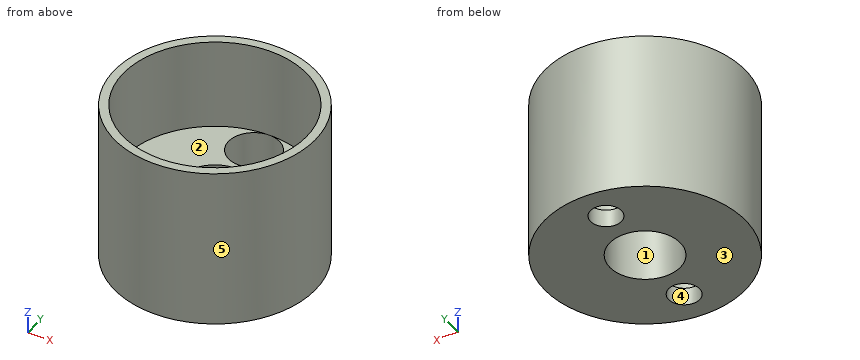
Autodesk Inventor part; units mm, degrees
ref_plane "Work Plane1" through (-9.0805, -9.0805, 27.1559) normal (0, 0, -1) x (0.0062, 1, 0)
ref_plane "YZ Plane" through (0, 0, 0) normal (1, 0, 0) x (0, 1, 0)
ref_plane "XZ Plane" through (0, 0, 0) normal (0, 1, 0) x (-1, 0, 0)
sketch "Sketch1" plane through (0, 0, 0) normal (0, 0, 1) x (1, 0, 0)
  circle A0 centre (0, 0) radius 9.025
  dimension "d0" = 18.05
extrude "Extrusion1" add sketch "Sketch1" along normal blind 6.35
sketch "Sketch4" plane through (0, 0, 6.35) normal (0, 0, 1) x (1, 0, 0)
  circle A0 centre (0, 0) radius 3.175
  dimension "d6" = 6.35
sketch "Sketch6" plane through (0, 0, 6.35) normal (0, 0, 1) x (1, 0, 0)
  circle A0 centre (0, 0) radius 9.025
  circle A1 centre (0, 0) radius 8.2312
  circle A2 centre (0, 0) radius 9.025
  dimension "d11" = 0.7937
ref_plane "Work Plane1" through (-9.0805, -9.0805, 27.1559) normal (0, 0, -1) x (0.0062, 1, 0)
extrude "Extrusion3" add sketch "Sketch6" along normal up to surface (20.8059 mm away)
sketch "Sketch7" plane through (0, 0, 6.35) normal (0, 0, 1) x (1, 0, 0)
  circle A0 centre (0, 5.9436) radius 1.397
  circle A1 centre (0, -5.9436) radius 1.397
  circle A2 centre (0, 0) radius 8.2312
  dimension "d20" = 2.794
  dimension "d21" = 2.794
  dimension "d22" = 5.9436
  dimension "d23" = 5.9436
extrude "Extrusion4" cut sketch "Sketch7" against normal blind 25.4 contours A0 | A1
sketch "Sketch8" plane through (0, 0, 6.35) normal (0, 0, 1) x (1, 0, 0)
  circle A0 centre (0, 5.9436) radius 2.286
  circle A1 centre (0, -5.9436) radius 2.286
  circle A2 centre (0, 5.9436) radius 1.397
  circle A3 centre (0, -5.9436) radius 1.397
  point P0 (0, 0)
  dimension "d16" = 4.572
  dimension "d17" = 4.572
extrude "Extrusion5" cut sketch "Sketch8" against normal blind 4.7625 contours A0 | A1 | A2 | A3
extrude "Extrusion6" cut sketch "Sketch4" against normal blind 25.4
sketch "Sketch9" plane through (0, 0, 27.1559) normal (0, 0, 1) x (1, 0, 0)
  circle A0 centre (27.8867, -20.1987) radius 65.8542
  point P0 (0, 0)
extrude "Extrusion7" cut sketch "Sketch9" against normal blind 12.7
properties part number "Cap Cap no LED"
Could you check a few things on this model? Use its own coordinates, in mm. Face numbers are marked on the shaded views. A direction names the side the tool comes from. Coordinates: 2 decimals unless noted, no trailing zeros. Write each loop counter-clockwise with the first axis right and the second up, starting at its lowest first coordinate (ties: lowest second). Pieces come first, ordered by that corner, then holes. Notation, with made-up numbers: (76.25, 77.5) -> (128.25, 77.5) arc R33 cw to (128.25, 105.5) -> close; hole circle Ø1 at (14, 42.25). An arc over 180 degrees is marked (long way). Write item = value, one per line. Start each with the question number.
(1) Will these pins go through, and if not, where does the flat tip stop? pin 1 (3 mm diameter, centred on y = 3, z = 5, fed in from +X); pin 2 (2.5 mm diameter, centred on x = 0, y = -5.94, fed in from +Z); pin 3 (3.5 mm diameter, centred on x = -0.5, y = -6.5, fed in from +Z); pin 4 (1.5 mm diameter, centred on x = 7, z = 5, fed in from -Y).
(2) We'd pull the mould along X, two halves only. Please class the marked faces 3, 4 and 5: released by +X, released by -X, zero draft, split by the parting line, or undercut.
(3) I want a section at A-A (y = 0). Please give me the cut outline in (x, z) (3 decimals).
(4) I want a section at B-B (x = 0). Give the number of separate pieces and of enclosed holes in the cut face, plus the area to 3 significant figures.
(5) I want a section at D-D (y = -5). Please give me the cut outline in (x, z), plus the area to 3 significant figures.
(6) Which directions (+Z, -Z, +X, -X, +Y, -Y) give clear straight access to the entire face, cutting with the end or side of a thin tool? Please do the marked faces 1 and 2.
(7) I want a section at C-C (z = 7). Please give me the cut outline in (x, y) (3 decimals), plus the area to 3 significant figures.
(8) I need wall thicknesses on line 1 (Y direction, x = 0, z = 5) (3 decimals); line 2 (Y direction, x = 0, z = 9) (3 decimals); line 3 (X direction, y = -0.25, z = 10.5). Which ranges of each line are inside material? Lowest first, please. Write a range as [from, to].
Result set:
q1.pin_1 = 8.9
q1.pin_2 = through
q1.pin_3 = 14.46
q1.pin_4 = -6.51
q2.face_3 = zero draft
q2.face_4 = undercut
q2.face_5 = split by the parting line
q3.outline = (-9.025, 0) -> (-3.175, 0) -> (-3.175, 6.35) -> (-8.231, 6.35) -> (-8.231, 14.456) -> (-9.025, 14.456) -> close; (3.175, 0) -> (9.025, 0) -> (9.025, 14.456) -> (8.231, 14.456) -> (8.231, 6.35) -> (3.175, 6.35) -> close
q4.separate_pieces = 4
q4.enclosed_holes = 0
q4.area = 34.7 mm2
q5.outline = (-7.51, 0) -> (-1.03, 0) -> (-1.03, 1.59) -> (-2.08, 1.59) -> (-2.08, 6.35) -> (-6.54, 6.35) -> (-6.54, 14.46) -> (-7.51, 14.46) -> close; (1.03, 0) -> (7.51, 0) -> (7.51, 14.46) -> (6.54, 14.46) -> (6.54, 6.35) -> (2.08, 6.35) -> (2.08, 1.59) -> (1.03, 1.59) -> close
q5.area = 88.1 mm2
q6.face_1 = +Z, -Z
q6.face_2 = +Z
q7.outline = circle Ø18.05 at (0, 0); hole circle Ø16.462 at (0, 0)
q7.area = 43.0 mm2
q8.line_1 = [-9.025, -8.23], [-3.658, -3.175], [3.175, 3.658], [8.23, 9.025]
q8.line_2 = [-9.025, -8.231], [8.231, 9.025]
q8.line_3 = [-9.02, -8.23], [8.23, 9.02]
